from build123d import *

# Parameters (mm, degrees)
F0_R     = 45
F0_R_2   = 2
F1_DEPTH = 1.5
F2_DEPTH = 35


# Not quite as in the source:
# - a fillet or chamfer that OpenCascade refuses, or shapes differently, is made with other operations: its cross-section is extruded or revolved along the edge and cut away or added


with BuildPart() as f1:
    # F0 (on Top) → F1 (new body)
    with BuildSketch(Plane.XY):
        Circle(F0_R)
        Circle(F0_R_2, mode=Mode.SUBTRACT)
    extrude(amount=F1_DEPTH)

    # F0 (on Top) → F2 (join)
    with BuildSketch(Plane.XY):
        Circle(F0_R_2)
    extrude(amount=F2_DEPTH)

    # F3: fillet of radius 2 on 1 edges, made by hand

    # F3_s1 → F3_t2 (revolve, cut)
    with BuildSketch(Plane.XZ):
        with BuildLine():
            ThreePointArc((45, 1.5), (44.2882531983, 0.4188611699), (43.0635083269, 0))
            Line((43.0635083269, 0), (45, 0))
            Line((45, 0), (45, 1.5))
        make_face()
    revolve(axis=Axis((0, 0, 0), (0, 0, 1)), mode=Mode.SUBTRACT)


solid = f1.part
Could you check a few things on this model? Use its own coordinates, in mm. A direction names the side the tool comes from. Give positions to 0.01 mm unless a question says otherwise; leave off trailing zeros. Write each loop counter-clockwise with the first axis right and the second up, starting at its lowest first coordinate (ties: lowest second). Pieces come first, ordered by that corner, then holes. Notation, with made-up numbers: (48, 20) -> (77, 20) arc R15 cw to (77, 24) -> close; hole circle Ø7 at (-24, 30.5). An arc over 180 degrees is marked (long way). Answer as a JSON object with one key per item and string values.
Q1. Please list where these lines run through material, in increasing order: L1, parallel to Z at x = 36, y = -17; L2, parallel to Y at x = -1, z = 29.5; L3, parallel to Y at x = 1.5, z = 27.
Taken from the geometry:
{"L1": "z = 0 to 1.5", "L2": "y = -1.73 to 1.73", "L3": "y = -1.32 to 1.32"}
Q2. Which directions (+Z, -Z, +X, -X, +Y, -Y) give clear straight access to the entire face, cutting with the end or side of a thin tool? Please do faces 1 (the flat face through (0, 0, 35)), 2 (the cylindrical face through (0, -2, 18)).
Taken from the geometry:
{"face 1": "+Z, +X, -X, +Y, -Y", "face 2": "+Z"}
Q3. Suppose I cut it at C-C on z = 6.5. Write out the boundary of the cut face in (x, y), then the cut area to 3 significant figures.
Taken from the geometry:
{"outline": "circle Ø4 at (0, 0)", "area": "12.6 mm²"}
Q4. Will these pins go through, and if not, where does the flat tip stop? pin 1 Ø12 at (x, y) = (28, 27.5) entering from +Z; pin 2 Ø12 at (y, z) = (1, 10) entering from +X.
Taken from the geometry:
{"pin 1": "stops at z = 1.5", "pin 2": "stops at x = 2"}
Q5. Suppose I cut it at A-A on x = 0. Write out the boundary of the cut face in (y, z).
Taken from the geometry:
{"outline": "(-45, 1.5) arc R2 ccw to (-43.06, 0) -> (43.06, 0) arc R2 ccw to (45, 1.5) -> (2, 1.5) -> (2, 35) -> (-2, 35) -> (-2, 1.5) -> close"}
